CAD build for the part. Positions are in the model's coordinates, mm. Face numbers are marked on the shaded views. Give positions to 0.01 mm unless a question says otherwise; leave off trailing zeros. Write each loop counter-clockwise with the first axis right and the second up, starting at its lowest first coordinate (ties: lowest second). Pieces come first, ordered by that corner, then holes. Notation, with made-up numbers: (69.25, -12) -> (99.25, -12) arc R28 ccw to (99.25, 8) -> close; hole circle Ø3 at (33, -6). An arc over 180 degrees is marked (long way). Answer in a Markdown table with one row per item. Add a question column.
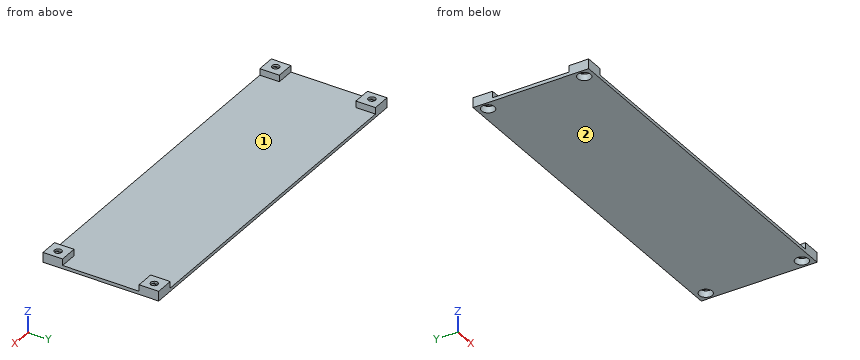
```python
from build123d import *
from build123d.topology import SkipClean

# Parameters (mm, degrees)
SKETCH1_W               = 112
SKETCH1_H               = 35.5
BOSS_EXTRUDE1_DEPTH     = 1
SKETCH2_W               = 6
SKETCH2_H               = 6
BOSS_EXTRUDE2_DEPTH     = 2
SKETCH3_R               = 1.1
CUT_EXTRUDE1_DEPTH      = 59.822295943
SKETCH4_R               = 2
CUT_EXTRUDE2_DEPTH      = 2
CUT_EXTRUDE3_DEPTH      = 0.2
SKETCH6_W               = 2.2
SKETCH6_H               = 2.2
CUT_EXTRUDE4_DEPTH      = 0.2
MIRROR2_COPY_1_DEPTH    = 0.2
MIRROR2_COPY_2_SKETCH_W = 2.2
MIRROR2_COPY_2_SKETCH_H = 2.2
MIRROR2_COPY_2_DEPTH    = 0.2
SKETCH7_W               = 0.4
SKETCH7_H               = 35.5
CUT_EXTRUDE5_DEPTH      = 59.822295943


with BuildPart() as part:
    # Sketch1 → Boss-Extrude1 (new body)
    with BuildSketch(Plane.XY):
        Rectangle(SKETCH1_W, SKETCH1_H)
    extrude(amount=BOSS_EXTRUDE1_DEPTH)

    # Sketch2 → Boss-Extrude2 (add)
    with BuildSketch(Plane.XY.offset(1)):
        with Locations((-53, 14.75)):
            Rectangle(SKETCH2_W, SKETCH2_H)
        with Locations((-53, -14.75)):
            Rectangle(SKETCH2_W, SKETCH2_H)
        with Locations((53, -14.75)):
            Rectangle(SKETCH2_W, SKETCH2_H)
        with Locations((53, 14.75)):
            Rectangle(SKETCH2_W, SKETCH2_H)
    extrude(amount=BOSS_EXTRUDE2_DEPTH)

    # Sketch3 → Cut-Extrude1 (cut, through all)
    with BuildSketch(Plane.XY.offset(3)):
        with Locations((-53, 14.75)):
            Circle(SKETCH3_R)
        with Locations(Location((-53, -14.75, 0), (0, 0, 180))):
            Circle(SKETCH3_R)
        with Locations((53, -14.75)):
            Circle(SKETCH3_R)
        with Locations(Location((53, 14.75, 0), (0, 0, 180))):
            Circle(SKETCH3_R)
    extrude(amount=-CUT_EXTRUDE1_DEPTH, mode=Mode.SUBTRACT)

    # Sketch4 → Cut-Extrude2 (cut)
    with BuildSketch(Plane(origin=(0, 0, 0), x_dir=(-1, 0, 0), z_dir=(0, 0, -1))):
        with Locations((-53, 14.75)):
            Circle(SKETCH4_R)
        with Locations((-53, -14.75)):
            Circle(SKETCH4_R)
        with Locations((53, 14.75)):
            Circle(SKETCH4_R)
        with Locations((53, -14.75)):
            Circle(SKETCH4_R)
    extrude(amount=-CUT_EXTRUDE2_DEPTH, mode=Mode.SUBTRACT)

    # Sketch5 → Cut-Extrude3 (cut)
    with SkipClean():  # the faces are left unmerged after this step: merging them gives an invalid solid
        with BuildSketch(Plane(origin=(0, 0, 2), x_dir=(-1, 0, 0), z_dir=(0, 0, -1))):
            with BuildLine():
                Line((-54.1, 13.079670691), (-54.1, 16.420329309))
                ThreePointArc((-54.1, 16.420329309), (-53, 16.75), (-51.9, 16.420329309))
                Line((-51.9, 16.420329309), (-51.9, 13.079670691))
                ThreePointArc((-51.9, 13.079670691), (-53, 12.75), (-54.1, 13.079670691))
            make_face()
        cut_extrude3 = extrude(amount=-CUT_EXTRUDE3_DEPTH, mode=Mode.SUBTRACT)

    # Sketch6 → Cut-Extrude4 (cut)
    with SkipClean():  # the faces are left unmerged after this step: merging them gives an invalid solid
        with BuildSketch(Plane(origin=(0, 0, 2.2), x_dir=(-1, 0, 0), z_dir=(0, 0, -1))):
            with Locations((-53, 14.75)):
                Rectangle(SKETCH6_W, SKETCH6_H)
        cut_extrude4 = extrude(amount=-CUT_EXTRUDE4_DEPTH, mode=Mode.SUBTRACT)

    # Mirror1: Cut-Extrude3, Cut-Extrude4 across plane
    with SkipClean():  # the faces are left unmerged after this step: merging them gives an invalid solid
        add(cut_extrude3.mirror(Plane(origin=(0, 0, 0), x_dir=(0, 0, 1), z_dir=(1, 0, 0))), mode=Mode.SUBTRACT)
        add(cut_extrude4.mirror(Plane(origin=(0, 0, 0), x_dir=(0, 0, 1), z_dir=(1, 0, 0))), mode=Mode.SUBTRACT)

    # Mirror2: Cut-Extrude3, Cut-Extrude4 across plane
    with SkipClean():  # the faces are left unmerged after this step: merging them gives an invalid solid
        add(cut_extrude3.mirror(Plane.ZX), mode=Mode.SUBTRACT)
        add(cut_extrude4.mirror(Plane.ZX), mode=Mode.SUBTRACT)

    # Mirror2 copy 1 sketch → Mirror2 copy 1 (cut)
    with SkipClean():  # the faces are left unmerged after this step: merging them gives an invalid solid
        with BuildSketch(Plane(origin=(0, 0, 2), x_dir=(1, 0, 0), z_dir=(0, 0, -1))):
            with BuildLine():
                Line((-54.1, 13.079670691), (-54.1, 16.420329309))
                ThreePointArc((-54.1, 16.420329309), (-53, 16.75), (-51.9, 16.420329309))
                Line((-51.9, 16.420329309), (-51.9, 13.079670691))
                ThreePointArc((-51.9, 13.079670691), (-53, 12.75), (-54.1, 13.079670691))
            make_face()
        extrude(amount=-MIRROR2_COPY_1_DEPTH, mode=Mode.SUBTRACT)

    # Mirror2 copy 2 sketch → Mirror2 copy 2 (cut)
    with SkipClean():  # the faces are left unmerged after this step: merging them gives an invalid solid
        with BuildSketch(Plane(origin=(0, 0, 2.2), x_dir=(1, 0, 0), z_dir=(0, 0, -1))):
            with Locations((-53, 14.75)):
                Rectangle(MIRROR2_COPY_2_SKETCH_W, MIRROR2_COPY_2_SKETCH_H)
        extrude(amount=-MIRROR2_COPY_2_DEPTH, mode=Mode.SUBTRACT)

    # Sketch7 → Cut-Extrude5 (cut, through all)
    with SkipClean():  # the faces are left unmerged after this step: merging them gives an invalid solid
        with BuildSketch(Plane(origin=(0, 0, 0), x_dir=(-1, 0, 0), z_dir=(0, 0, -1))):
            with Locations((-55.8, 0)):
                Rectangle(SKETCH7_W, SKETCH7_H)
            with Locations((55.8, 0)):
                Rectangle(SKETCH7_W, SKETCH7_H)
        extrude(amount=-CUT_EXTRUDE5_DEPTH, mode=Mode.SUBTRACT)


solid = part.part
```
Item 1: Mould opens along X. For the marked faces 1 and 2 say: released by +X, released by -X, zero draft, split by the parting line, or undercut.
Item 2: Slice it at B-B, the plane x = 37. List the corners of the cut face in (y, z), then the cut area to 3 significant figures.
Item 3: Drop a flat-ended pin along its axis: pin 1 Ø3 at (x, y) = (53, 14.75) entering from -Z. Give the stop position or say it passes through.
Item 4: Probe L1, parallel to Y at x = -53, z = 2.65; L2, parallel to X at y = 14.75, z = 0.75; L3, parallel to Y at x = 53, z = 1.55. List the from-to ranges inside material, lowest first. Write a range as from..to.
Item 5: Slice it at A-A, the plane y = 5. List the corners of the cut face in (x, z).
Answer key:
| question | item | result |
|---|---|---|
| 1 | face 1 | undercut |
| 1 | face 2 | zero draft |
| 2 | outline | (-17.75, 0) -> (17.75, 0) -> (17.75, 1) -> (-17.75, 1) -> close |
| 2 | area | 35.5 mm² |
| 3 | pin 1 | stops at z = 2 |
| 4 | L1 | y = -17.75..-15.85, -13.65..-11.75, 11.75..13.65, 15.85..17.75 |
| 4 | L2 | x = -55.6..-55, -51..51, 55..55.6 |
| 4 | L3 | y = -17.75..-16.75, -12.75..-11.75, 11.75..12.75, 16.75..17.75 |
| 5 | outline | (-55.6, 0) -> (55.6, 0) -> (55.6, 1) -> (-55.6, 1) -> close |
